Geometry check sheet. Reference: the model listing, model coordinates, mm. Face numbers are marked on the shaded views. A direction names the side the tool comes from. Round coordinates to 2 decimals unless told otherwise and drop trailing zeros. Loops run counter-clockwise (first coordinate to the right, second up) from the corner with the lowest first, then second, coordinate; pieces in that order, holes last. Notation, with made-up numbers: M 37,25.25 L 78,25.25 A5 cw 78,31.25 Z; hole C -34.75,58 d5. An arc over 180 degrees is marked long. Use one line per item in the form item = value. Start each with the question number.
1. Cross-section at A-A (y = 38.1). State how many separate pieces and enclosed holes the cut face has, then the cut area to 3 significant figures.
2. Set-up check for the marked faces 4 and 5: record each of +Z, -Z, +X, -X, +Y, -Y from which the full face is reachable in a straight line by a thin tool's end or side.
3. Go/stop test with flat-tipped pins: pin 1 (8 mm diameter, centred on y = 20.5, z = 19.5, fed in from -X); pin 2 (4 mm diameter, centred on x = 25.4, y = 12.7, fed in from +Z). Record where each tip stops, or that it passes through.
4. Material ranges on line 1 (Y direction, x = 12.7, z = 1.8); line 2 (X direction, y = 1.95, z = 12.7); line 3 (Z direction, x = 41, y = 24.5) (3 decimals), recorded low to high.
5. Cross-section at B-B (y = 29.5). Record the boundary of the cut face in (x, z) (3 decimals), then the cut area to 3 significant figures.
6. Draft check along Y on the marked faces 1, 2 and 3. Enter one of: pulls with the +Y half, pulls with the -Y half, needs draft (parallel to the pull), parting line crosses it, or undercut.
```python
from build123d import *

# Parameters (mm, degrees)
SKETCH1_W           = 50.8
SKETCH1_H           = 50.8
BOSS_EXTRUDE1_DEPTH = 25.4
SKETCH2_W           = 19.05
SKETCH2_H           = 44.45
CUT_EXTRUDE1_DEPTH  = 77.2
SKETCH3_R           = 2.5527
CUT_EXTRUDE2_DEPTH  = 77.2
SKETCH4_R           = 2.5527
CUT_EXTRUDE3_DEPTH  = 77.2


with BuildPart() as part:
    # Sketch1 → Boss-Extrude1 (new body)
    with BuildSketch(Plane.XY):
        with Locations((25.4, 25.4)):
            Rectangle(SKETCH1_W, SKETCH1_H)
    extrude(amount=BOSS_EXTRUDE1_DEPTH)

    # Sketch2 → Cut-Extrude1 (cut, through all)
    with BuildSketch(Plane(origin=(50.8, 0, 0), x_dir=(0, 0, -1), z_dir=(1, 0, 0))):
        with Locations((-12.7, 25.4)):
            Rectangle(SKETCH2_W, SKETCH2_H)
    extrude(amount=-CUT_EXTRUDE1_DEPTH, mode=Mode.SUBTRACT)

    # Sketch3 → Cut-Extrude2 (cut, through all)
    with BuildSketch(Plane(origin=(0, 50.8, 0), x_dir=(1, 0, 0), z_dir=(0, 1, 0))):
        with Locations(Location((12.7, -12.7, 0), (0, 0, 270))):
            Circle(SKETCH3_R)
        with Locations(Location((25.4, -12.7, 0), (0, 0, 270))):
            Circle(SKETCH3_R)
        with Locations(Location((38.1, -12.7, 0), (0, 0, 270))):
            Circle(SKETCH3_R)
    extrude(amount=-CUT_EXTRUDE2_DEPTH, mode=Mode.SUBTRACT)

    # Sketch4 → Cut-Extrude3 (cut, through all)
    with BuildSketch(Plane(origin=(0, 0, 0), x_dir=(-1, 0, 0), z_dir=(0, 0, -1))):
        with Locations((-38.1, 38.1)):
            Circle(SKETCH4_R)
        with Locations((-25.4, 38.1)):
            Circle(SKETCH4_R)
        with Locations((-12.7, 38.1)):
            Circle(SKETCH4_R)
        with Locations((-38.1, 12.7)):
            Circle(SKETCH4_R)
        with Locations((-25.4, 12.7)):
            Circle(SKETCH4_R)
        with Locations((-12.7, 12.7)):
            Circle(SKETCH4_R)
    extrude(amount=-CUT_EXTRUDE3_DEPTH, mode=Mode.SUBTRACT)


solid = part.part
```
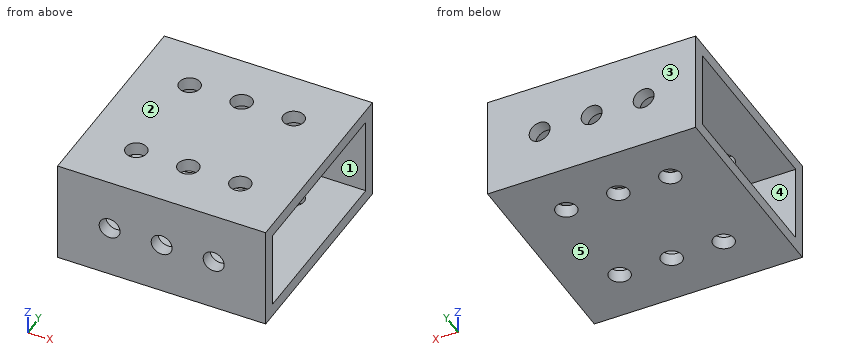
Reported:
q1.separate_pieces = 8
q1.enclosed_holes = 0
q1.area = 225 mm²
q2.face_4 = +X, -X
q2.face_5 = -Z, +X, -X, +Y, -Y
q3.pin_1 = 0
q3.pin_2 = through
q4.line_1 = 0 to 10.15, 15.25 to 35.55, 40.65 to 50.8
q4.line_2 = 0 to 10.15, 15.25 to 22.85, 27.95 to 35.55, 40.65 to 50.8
q4.line_3 = 0 to 3.175, 22.225 to 25.4
q5.outline = M 0,0 L 50.8,0 L 50.8,3.175 L 0,3.175 Z; M 0,22.225 L 50.8,22.225 L 50.8,25.4 L 0,25.4 Z
q5.area = 323 mm²
q6.face_1 = undercut
q6.face_2 = needs draft
q6.face_3 = pulls with the +Y half
